The listing builds one solid part. Answer for the finished solid, in the listing's coordinates (mm). Face numbers are marked on the shaded views. Give positions to 0.01 mm unless a question says otherwise; leave off trailing zeros. Write each loop counter-clockwise with the first axis right and the second up, starting at its lowest first coordinate (ties: lowest second). Pieces come first, ordered by that corner, then holes. Notation, with made-up numbers: (-16, 23.5) - (33, 23.5) arc R14 cw to (33, 35.5) - close; hole circle Ø2 at (4.5, 25). An arc over 180 degrees is marked (long way). Write each question's results on one line, items separated by ' | '. Start each with the question number.
Q1. For a pull along X with two mould halves and no side action, classify the marked faces 1 and 2 as pulls with the +X half, pulls with the -X half, needs draft (parallel to the pull), parting line crosses it, or undercut.
Q2. Section A-A (x = 11) is taken. Determine the outline of the cut face in (y, z).
Q3. Section C-C (x = 43.5) is taken. Determine the outline of the cut face in (y, z).
Q4. Find the intervals of material crossed by probe 1 along Z at (x, y) = (55.5, 0.45); probe 2 along Z at (x, y) = (16, 0.3); probe 3 along X at (y, z) = (3.75, -14), in increasing order.
Q5. Flat-ended cylindrical pins translate along their axes: pin 1 Ø0.6 at (x, y) = (55, 2.5) entering from -Z; pin 2 Ø2.5 at (x, z) = (36, -28.86) entering from -Y; pin 3 Ø0.8 at (y, z) = (0.5, -9) entering from +X; pin 4 Ø0.6 at (x, y) = (15.5, 2) entering from +Z. Find the tip coordinate at first contact, or state that the pin passes through.
Q6. Section B-B (z = -13) is taken. Determine the outline of the cut face in (x, y).
```python
from build123d import *

# Parameters (mm, degrees)
SKETCH1_R           = 1.5
BOSS_EXTRUDE1_DEPTH = 1.5
SKETCH2_W           = 24
SKETCH2_H           = 16
BOSS_EXTRUDE2_DEPTH = 1.3
SKETCH3_W           = 15
SKETCH3_H           = 12
BOSS_EXTRUDE3_DEPTH = 2.2
SKETCH4_R           = 1
CUT_EXTRUDE1_DEPTH  = 2.5
SKETCH5_W           = 6
SKETCH5_H           = 8
BOSS_EXTRUDE4_DEPTH = 2.4
FILLET1_R           = 0.5


with BuildPart() as part:
    # Sketch1 → Boss-Extrude1 (new body)
    with BuildSketch(Plane(origin=(0, 0, 0), x_dir=(1, 0, 0), z_dir=(0, 1, 0))):
        Polygon((0, 30), (1, 31), (57, 31), (58, 30), (58, 1), (57, 0), (1, 0), (0, 1), align=None)
        with Locations((2.5, 28.5)):
            Circle(SKETCH1_R, mode=Mode.SUBTRACT)
        with Locations((2.5, 2.5)):
            Circle(SKETCH1_R, mode=Mode.SUBTRACT)
        with Locations((55.5, 28.5)):
            Circle(SKETCH1_R, mode=Mode.SUBTRACT)
        with Locations((55.5, 2.5)):
            Circle(SKETCH1_R, mode=Mode.SUBTRACT)
    extrude(amount=BOSS_EXTRUDE1_DEPTH)

    # Sketch2 → Boss-Extrude2 (add)
    with BuildSketch(Plane(origin=(0, 1.5, 0), x_dir=(1, 0, 0), z_dir=(0, 1, 0))):
        with Locations((12, 15.5)):
            Rectangle(SKETCH2_W, SKETCH2_H)
    extrude(amount=BOSS_EXTRUDE2_DEPTH)

    # Sketch3 → Boss-Extrude3 (add)
    with BuildSketch(Plane(origin=(0, 2.8, 0), x_dir=(1, 0, 0), z_dir=(0, 1, 0))):
        with Locations((15.5, 15.5)):
            Rectangle(SKETCH3_W, SKETCH3_H)
    extrude(amount=BOSS_EXTRUDE3_DEPTH)

    # Sketch4 → Cut-Extrude1 (cut, through all)
    with BuildSketch(Plane(origin=(0, 1.5, 0), x_dir=(1, 0, 0), z_dir=(0, 1, 0))):
        with Locations((11, 2.139657304)):
            Circle(SKETCH4_R)
        with Locations((13.5, 2.139657304)):
            Circle(SKETCH4_R)
        with Locations((16, 2.139657304)):
            Circle(SKETCH4_R)
        with Locations((18.5, 2.139657304)):
            Circle(SKETCH4_R)
        with Locations((21, 2.139657304)):
            Circle(SKETCH4_R)
        with Locations((23.5, 2.139657304)):
            Circle(SKETCH4_R)
        with Locations((26, 2.139657304)):
            Circle(SKETCH4_R)
        with Locations((28.5, 2.139657304)):
            Circle(SKETCH4_R)
        with Locations((31, 2.139657304)):
            Circle(SKETCH4_R)
        with Locations((33.5, 2.139657304)):
            Circle(SKETCH4_R)
        with Locations((36, 2.139657304)):
            Circle(SKETCH4_R)
        with Locations((38.5, 2.139657304)):
            Circle(SKETCH4_R)
        with Locations((41, 2.139657304)):
            Circle(SKETCH4_R)
        with Locations((43.5, 2.139657304)):
            Circle(SKETCH4_R)
        with Locations((46, 2.139657304)):
            Circle(SKETCH4_R)
        with Locations((46, 28.860342696)):
            Circle(SKETCH4_R)
        with Locations((43.5, 28.860342696)):
            Circle(SKETCH4_R)
        with Locations((41, 28.860342696)):
            Circle(SKETCH4_R)
        with Locations((38.5, 28.860342696)):
            Circle(SKETCH4_R)
        with Locations((36, 28.860342696)):
            Circle(SKETCH4_R)
        with Locations((33.5, 28.860342696)):
            Circle(SKETCH4_R)
        with Locations((31, 28.860342696)):
            Circle(SKETCH4_R)
        with Locations((28.5, 28.860342696)):
            Circle(SKETCH4_R)
        with Locations((26, 28.860342696)):
            Circle(SKETCH4_R)
        with Locations((23.5, 28.860342696)):
            Circle(SKETCH4_R)
        with Locations((21, 28.860342696)):
            Circle(SKETCH4_R)
        with Locations((18.5, 28.860342696)):
            Circle(SKETCH4_R)
        with Locations((16, 28.860342696)):
            Circle(SKETCH4_R)
        with Locations((13.5, 28.860342696)):
            Circle(SKETCH4_R)
        with Locations((11, 28.860342696)):
            Circle(SKETCH4_R)
    extrude(amount=-CUT_EXTRUDE1_DEPTH, mode=Mode.SUBTRACT)

    # Sketch5 → Boss-Extrude4 (add)
    with BuildSketch(Plane(origin=(0, 1.5, 0), x_dir=(1, 0, 0), z_dir=(0, 1, 0))):
        with Locations((56, 15.5)):
            Rectangle(SKETCH5_W, SKETCH5_H)
    extrude(amount=BOSS_EXTRUDE4_DEPTH)

    # Fillet1
    fillet1_edges = [part.edges().sort_by_distance(p)[0] for p in [
        (56, 3.9, -11.5),
        (56, 3.9, -19.5),
    ]]
    fillet(fillet1_edges, radius=FILLET1_R)


solid = part.part
```
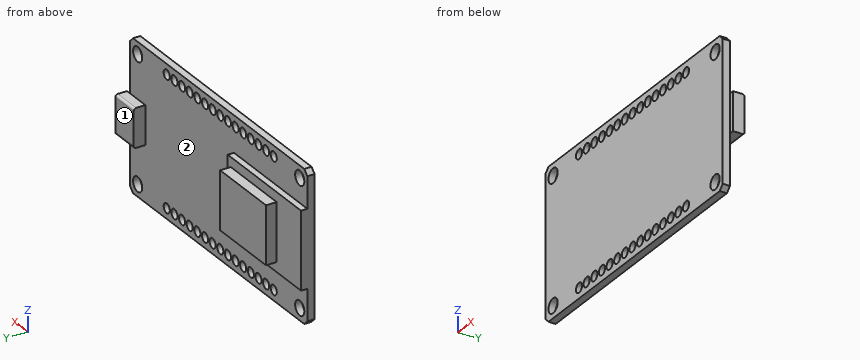
Answers below:
1) face 1: needs draft | face 2: undercut
2) outline: (0, -31) - (1.5, -31) - (1.5, -29.86) - (0, -29.86) - close; (0, -27.86) - (1.5, -27.86) - (1.5, -23.5) - (2.8, -23.5) - (2.8, -21.5) - (5, -21.5) - (5, -9.5) - (2.8, -9.5) - (2.8, -7.5) - (1.5, -7.5) - (1.5, -3.14) - (0, -3.14) - close; (0, -1.14) - (1.5, -1.14) - (1.5, 0) - (0, 0) - close
3) outline: (0, -31) - (1.5, -31) - (1.5, -29.86) - (0, -29.86) - close; (0, -27.86) - (1.5, -27.86) - (1.5, -3.14) - (0, -3.14) - close; (0, -1.14) - (1.5, -1.14) - (1.5, 0) - (0, 0) - close
4) probe 1: z = -31 to -30, -27 to -4, -1 to 0 | probe 2: z = -31 to -29.86, -27.86 to -3.14, -1.14 to 0 | probe 3: x = 8 to 23, 53 to 59
5) pin 1: stops at z = -19.5 | pin 2: stops at y = 0 | pin 3: stops at x = 58 | pin 4: stops at z = -7.5
6) outline: (0, 0) - (58, 0) - (58, 1.5) - (59, 1.5) - (59, 3.9) - (53, 3.9) - (53, 1.5) - (24, 1.5) - (24, 2.8) - (23, 2.8) - (23, 5) - (8, 5) - (8, 2.8) - (0, 2.8) - close
